```python
from build123d import *

# Parameters (mm, degrees)
F1_DEPTH = 63.5
F2_DEPTH = 25.4
F3_DEPTH = 6.35
F5_R     = 6.35


with BuildPart() as f1:
    # F0 (on Front) → F1 (new body, symmetric)
    with BuildSketch(Plane.XZ):
        Polygon((41.275, -9.525), (41.275, 9.525), (22.225, 9.525), (-41.275, 9.525), (-41.275, -9.525), align=None)
    extrude(amount=F1_DEPTH, both=True)

    # F0 (on Front) → F2 (join, symmetric)
    with BuildSketch(Plane.XZ):
        Polygon((60.325, 61.9125), (60.325, 42.8625), (85.725, 42.8625), (85.725, 52.3875), (85.725, 61.9125), align=None)
        with BuildLine():
            Line((22.225, 9.525), (41.275, 9.525))
            Line((41.275, 9.525), (41.275, 26.9875))
            ThreePointArc((41.275, 26.9875), (45.92468, 38.21282), (57.15, 42.8625))
            Line((57.15, 42.8625), (60.325, 42.8625))
            Line((60.325, 42.8625), (60.325, 61.9125))
            Line((60.325, 61.9125), (57.15, 61.9125))
            add(Edge.make_bspline(
                [(56.128748, 61.897565), (56.46798, 61.902911), (56.808396, 61.907889), (57.15, 61.9125)],
                knots=[110.923942, 110.923942, 110.923942, 110.923942, 111.498569, 111.498569, 111.498569, 111.498569], degree=3))
            ThreePointArc((56.128748, 61.897565), (32.09583, 51.319458), (22.225, 26.9875))
            Line((22.225, 26.9875), (22.225, 9.525))
        make_face()
    extrude(amount=F2_DEPTH, both=True)

    # F0 (on Front) → F3 (join, symmetric)
    with BuildSketch(Plane.XZ):
        with BuildLine():
            Line((-41.275, 9.525), (22.225, 9.525))
            Line((22.225, 9.525), (22.225, 26.9875))
            ThreePointArc((22.225, 26.9875), (32.09583, 51.319458), (56.128748, 61.897565))
            add(Edge.make_bspline(
                [(-41.275, 9.525), (-30.753714, 46.112992), (-9.355641, 60.865587), (56.128748, 61.897565)],
                knots=[0, 0, 0, 0, 110.923942, 110.923942, 110.923942, 110.923942], degree=3))
        make_face()
    extrude(amount=F3_DEPTH, both=True)

    # F0 (on Front) → F4 (revolve)
    with BuildSketch(Plane.XZ):
        Polygon((85.725, 52.3875), (85.725, 42.8625), (85.725, 38.1), (111.125, 38.1), (111.125, 66.675), (85.725, 66.675), (85.725, 61.9125), align=None)
    revolve(axis=Axis((85.725, 0, 59.53125), (0, 0, 1)))

    # F5
    f5_edges = [f1.edges().sort_by_distance(p)[0] for p in [
        (41.275, -63.5, 0),
        (-41.275, -63.5, 0),
        (41.275, 63.5, 0),
        (-41.275, 63.5, 0),
    ]]
    fillet(f5_edges, radius=F5_R)


solid = f1.part
```
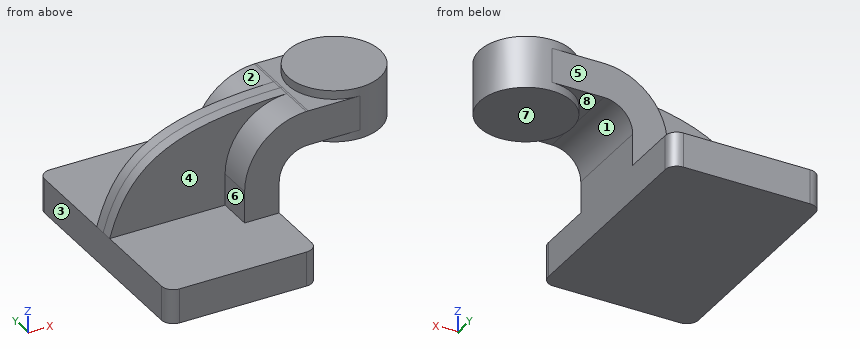
Model file for the job. Use its own axes, mm. Face numbers are marked on the shaded views. A direction names the side the tool comes from. Give positions to 0.01 mm unless a question says otherwise; leave off trailing zeros. Write each loop counter-clockwise with the first axis right and the second up, starting at its lowest first coordinate (ties: lowest second). Pieces come first, ordered by that corner, then holes. Notation, with made-up numbers: (-5.75, 64.25) - (39.25, 64.25) arc R13 ccw to (39.25, 88.25) - close; hole circle Ø1 at (23, 59). An arc over 180 degrees is marked (long way). One line per question, with ' | ' between items. Start each with the question number.
(1) Two-plate mould, pull along X, no slides. Class the marked faces 6, 7 and 8: +X half, -X half, draft (parallel to the pull), parting line (faces both ways), or undercut.
(2) Slice it at A-A on z = 2. Write the cut outline in (x, y) (3 decimals).
(3) Slice it at D-D on x = 96.5. Write the cut outline in (y, z) (3 decimals), plus the area to 3 significant figures.
(4) Slice it at C-C on y = 48.5. Write the cut outline in (x, z) (3 decimals).
(5) Pin check, flat tips, straight feed: P1, Ø12, axis at y = -29, z = 0, coming from the +X side (3 decimals); P2, Ø15.5, axis at x = 9, z = 35.5, coming from the +Y side; P3, Ø15.5, axis at x = -9, z = 25, coming from the -Y side. Stop position of each tip, or through.
(6) 3-axis set-ups, long thin cutter, end or side, ignore diameter. For the marked faces 1, 2, 3, 4 and 5: which of +Z, -Z, +X, -X, +Y, -Y reach the whole face in a straight line?
(7) Wall check: line 1 along Z through (x, y) = (27.5, 51) (3 decimals); line 2 along Y through (x, z) = (36, 18); line 3 along X through (y, z) = (-8, -3.5) (3 decimals). Give the ranges that are in metal, low to high. Write a range as from..to.
(8) Slice it at B-B on x = 72. Write the cut outline in (y, z) (1 decimal).
Results below:
1) face 6: -X half | face 7: draft | face 8: undercut
2) outline: (-41.275, -57.15) arc R6.35 ccw to (-34.925, -63.5) - (34.925, -63.5) arc R6.35 ccw to (41.275, -57.15) - (41.275, 57.15) arc R6.35 ccw to (34.925, 63.5) - (-34.925, 63.5) arc R6.35 ccw to (-41.275, 57.15) - close
3) outline: (-23.001, 38.1) - (23.001, 38.1) - (23.001, 66.675) - (-23.001, 66.675) - close | area: 1,310 mm^2
4) outline: (-41.275, -9.525) - (41.275, -9.525) - (41.275, 9.525) - (-41.275, 9.525) - close
5) P1: x = 41.275 | P2: y = 6.35 | P3: y = -6.35
6) face 1: -Z, +Y, -Y | face 2: +Z, -X, +Y | face 3: +Z, -Z, -X, +Y, -Y | face 4: +Z, -X, -Y | face 5: +Z, +X, -X, +Y
7) line 1: -9.525..9.525 | line 2: -25.4..25.4 | line 3: -41.275..41.275
8) outline: (-25.4, 42.9) - (-21.4, 42.9) - (-21.4, 38.1) - (21.4, 38.1) - (21.4, 42.9) - (25.4, 42.9) - (25.4, 61.9) - (21.4, 61.9) - (21.4, 66.7) - (-21.4, 66.7) - (-21.4, 61.9) - (-25.4, 61.9) - close
